```python
from build123d import *

# Parameters (mm, degrees)
SKETCH1_R           = 8.2
BOSS_EXTRUDE1_DEPTH = 9.5
SKETCH2_R           = 6.25
CUT_EXTRUDE1_DEPTH  = 4
SKETCH3_R           = 2.5
CUT_EXTRUDE2_DEPTH  = 13.83471854


with BuildPart() as part:
    # Sketch1 → Boss-Extrude1 (new body)
    with BuildSketch(Plane(origin=(0, 0, 0), x_dir=(1, 0, 0), z_dir=(0, 1, 0))):
        with Locations(Location((0, 0, 0), (0, 0, 270))):
            Circle(SKETCH1_R)
    extrude(amount=BOSS_EXTRUDE1_DEPTH)

    # Sketch2 → Cut-Extrude1 (cut)
    with BuildSketch(Plane(origin=(0, 9.5, 0), x_dir=(1, 0, 0), z_dir=(0, 1, 0))):
        with Locations(Location((0, 0, 0), (0, 0, 270))):
            Circle(SKETCH2_R)
    extrude(amount=-CUT_EXTRUDE1_DEPTH, mode=Mode.SUBTRACT)

    # Sketch3 → Cut-Extrude2 (cut, through all)
    with BuildSketch(Plane(origin=(0, 5.5, 0), x_dir=(1, 0, 0), z_dir=(0, 1, 0))):
        with Locations(Location((0, 0, 0), (0, 0, 270))):
            Circle(SKETCH3_R)
    extrude(amount=-CUT_EXTRUDE2_DEPTH, mode=Mode.SUBTRACT)


solid = part.part
```
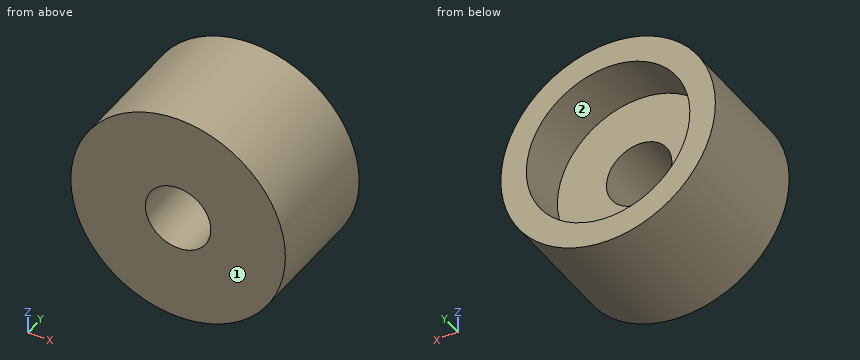
Geometry: final body of the model. Coordinates: model frame, mm. Face numbers are marked on the shaded views. A direction names the side the tool comes from. Coordinates: 2 decimals unless noted, no trailing zeros. Order: outer loops, then holes, each group sorted by start corner. A loop starts at its lowest first (then second) coordinate and runs counter-clockwise, first axis right, second up. Notation, with made-up numbers: M 46,14.5 L 65,14.5 A7 ccw 65,26.5 Z; hole C 76.25,89 d6. An arc over 180 degrees is marked long. Answer as CSV lines item,"result".
Q1. Section B-B on z = 0. Return the cut outline in (x, y), and give its area (3 significant figures).
Answers:
outline,"M -8.2,0 L -2.5,0 L -2.5,5.5 L -6.25,5.5 L -6.25,9.5 L -8.2,9.5 Z; M 2.5,0 L 8.2,0 L 8.2,9.5 L 6.25,9.5 L 6.25,5.5 L 2.5,5.5 Z"
area,"78.3 mm^2"
Q2. Section C-C on y = 1. Return the cut outline in (x, z).
Answers:
outline,"C 0,0 d16.4; hole C 0,0 d5"
Q3. Section D-D on z = -2.75. Return the cut outline in (x, y), and give its area (3 significant figures).
Answers:
outline,"M -7.73,0 L 7.73,0 L 7.73,9.5 L 5.61,9.5 L 5.61,5.5 L -5.61,5.5 L -5.61,9.5 L -7.73,9.5 Z"
area,"102 mm^2"
Q4. First-contact query: P1, Ø1.5, axis at x = 6, y = 6.5, coming from the -Z side; P2, Ø6, axis at x = 0, z = 0, coming from the +Y side; P3, Ø1, axis at x = 5, y = 2, coming from the -Z side. Flat tips, straight axial feed; report the tip coordinate or a pass-through.
Answers:
P1,"stops at z = -6.3"
P2,"stops at y = 5.5"
P3,"stops at z = -6.85"
Q5. Set-up query: the marked faces 1 and 2. Return all of +Z, -Z, +X, -X, +Y, -Y with unobstructed straight access to the full face (end or side cutting, diameter ignored); none if empty.
Answers:
face 1,"+Z, -Z, +X, -X, -Y"
face 2,"+Y"
Q6. Line query: probe 1 along X at (y, z) = (4.3, 0); probe 2 along X at (y, z) = (7.6, 0); probe 3 along Y at (x, z) = (1, 6). Output: solid intervals per line, ascending. Write a range as [from, to].
Answers:
probe 1,"x = [-8.2, -2.5], [2.5, 8.2]"
probe 2,"x = [-8.2, -6.25], [6.25, 8.2]"
probe 3,"y = [0, 5.5]"
Q7. Section A-A on x = 0. Return the cut outline in (y, z).
Answers:
outline,"M 0,-8.2 L 9.5,-8.2 L 9.5,-6.25 L 5.5,-6.25 L 5.5,-2.5 L 0,-2.5 Z; M 0,2.5 L 5.5,2.5 L 5.5,6.25 L 9.5,6.25 L 9.5,8.2 L 0,8.2 Z"
